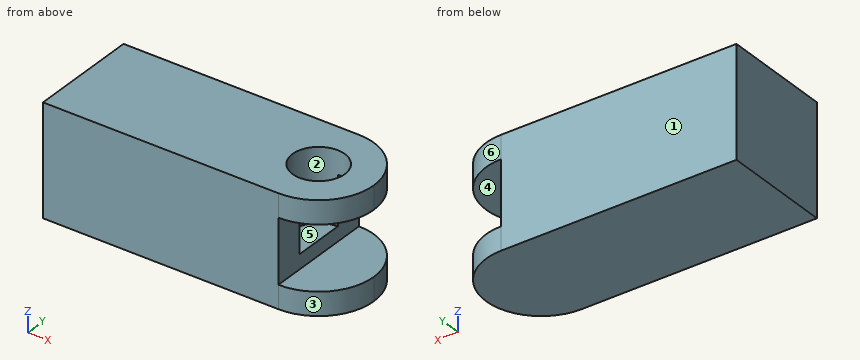
```python
from build123d import *

# Parameters (mm, degrees)
F0_W     = 100
F0_H     = 38
F1_DEPTH = 38
F2_R     = 18.99999
F3_R     = 9
F4_DEPTH = 25
F5_W     = 20.3221625665
F5_H     = 22
F6_DEPTH = 38.001


# Not quite as in the source:
# - a fillet or chamfer is up to 0.001 mm smaller than in the source, because OpenCascade refuses the exact size


with BuildPart() as f1:
    # F0 (on Top) → F1 (new body)
    with BuildSketch(Plane.XY):
        with Locations((50, 19)):
            Rectangle(F0_W, F0_H)
    extrude(amount=F1_DEPTH)

    # F2 (radius 19 in the source; OpenCascade refuses exactly that, so slightly less here)
    f2_edges = [f1.edges().sort_by_distance(p)[0] for p in [
        (100, 0, 19),
        (100, 38, 19),
    ]]
    fillet(f2_edges, radius=F2_R)

    # F3 (on face) → F4 (cut)
    with BuildSketch(Plane.XY.offset(38)):
        with Locations((81, 19)):
            Circle(F3_R)
    extrude(amount=-F4_DEPTH, mode=Mode.SUBTRACT)

    # F5 (on face) → F6 (cut, through all)
    with BuildSketch(Plane.XZ):
        with Locations((91.1610912833, 19)):
            Rectangle(F5_W, F5_H)
    extrude(amount=-F6_DEPTH, mode=Mode.SUBTRACT)


solid = f1.part
```
Build history of the part. All positions in model axes, mm. Face numbers are marked on the shaded views. A direction names the side the tool comes from. Coordinates: 2 decimals unless noted, no trailing zeros. Order: outer loops, then holes, each group sorted by start corner. A loop starts at its lowest first (then second) coordinate and runs counter-clockwise, first axis right, second up. Notation, with made-up numbers: (63.25, -17.75) -> (78.25, -17.75) arc R22 cw to (78.25, 7.25) -> close; hole circle Ø2 at (83, 24.5). An arc over 180 degrees is marked (long way). Answer in a Markdown table with one row per item. Add a question column.
Q1. Wall check: line 1 along X through (y, z) = (19, 32.5); line 2 along Y through (x, z) = (81, 32); line 3 along X through (y, z) = (19, 23.5). Give the ranges that are in metal, low to high. Write a range as [from, to].
Q2. Which spindle directions (+Z, -Z, +X, -X, +Y, -Y) get a long thin tool onto all of the face, cutting with end or side? Do the marked faces 4, 5 and 6. Say none if no direction does.
Q3. Drop a flat-ended pin along its axis: pin 1 (2.5 mm diameter, centred on x = 78, y = 15.5, fed in from +Z). Give the stop position or say it passes through.
Q4. Mould opens along X. For the marked faces 1, 2 and 3 say: +X half, -X half, draft (parallel to the pull), parting line (faces both ways), or undercut.
Q5. Band-saw the part on C-C, the plane z = 25. List the corners of the cut face in (x, y).
Q6. Band-saw the part on B-B, the plane y = 21. List the corners of the cut face in (x, z), then the cut area to 3 significant figures.
Q7. Band-saw the part on D-D, the plane y = 33.5. List the corners of the cut face in (x, z).
Answers follow:
| question | item | result |
|---|---|---|
| 1 | line 1 | [0, 72], [90, 100] |
| 1 | line 2 | [0, 10], [28, 38] |
| 1 | line 3 | [0, 72] |
| 2 | face 4 | +X, +Y, -Y |
| 2 | face 5 | +Z, +X |
| 2 | face 6 | +Z, -Z, +X, +Y |
| 3 | pin 1 | z = 13 |
| 4 | face 1 | draft |
| 4 | face 2 | undercut |
| 4 | face 3 | +X half |
| 5 | outline | (0, 0) -> (81, 0) -> (81, 10) arc R9 cw to (81, 28) -> (81, 38) -> (0, 38) -> close |
| 6 | outline | (0, 0) -> (99.89, 0) -> (99.89, 8) -> (81, 8) -> (81, 13) -> (72.23, 13) -> (72.23, 38) -> (0, 38) -> close; (89.77, 30) -> (99.89, 30) -> (99.89, 38) -> (89.77, 38) -> close |
| 6 | area | 3,090 mm^2 |
| 7 | outline | (0, 0) -> (93.28, 0) -> (93.28, 8) -> (81, 8) -> (81, 30) -> (93.28, 30) -> (93.28, 38) -> (0, 38) -> close |
